Read the model definition and answer for the solid it produces. Units are mm, in the model's axes. Round coordinates to 2 decimals unless told otherwise and drop trailing zeros. Write each loop counter-clockwise with the first axis right and the second up, starting at its lowest first coordinate (ties: lowest second). Pieces come first, ordered by that corner, then holes.
from build123d import *

# Parameters (mm, degrees)
SKETCH1_R           = 3.175
BOSS_EXTRUDE1_DEPTH = 41.275
CUT_EXTRUDE5_DEPTH  = 83.672025196
CUT_EXTRUDE8_DEPTH  = 15.875


with BuildPart() as part:
    # Sketch1 → Boss-Extrude1 (new, symmetric)
    with BuildSketch(Plane(origin=(0, 0, 0), x_dir=(1, 0, 0), z_dir=(0, 1, 0))):
        with Locations(Location((0, 0, 0), (0, 0, 270))):
            Circle(SKETCH1_R)
    extrude(amount=BOSS_EXTRUDE1_DEPTH, both=True)

    # Sketch2 → Cut-Extrude5 (cut, through all)
    with BuildSketch(Plane(origin=(0, 41.275, 0), x_dir=(1, 0, 0), z_dir=(0, 1, 0))):
        with BuildLine():
            Line((-2.549322464, 1.892506268), (2.530677536, 1.917366999))
            ThreePointArc((2.530677536, 1.917366999), (-0.015537771, 3.174961981), (-2.549322464, 1.892506268))
        make_face()
    extrude(amount=-CUT_EXTRUDE5_DEPTH, mode=Mode.SUBTRACT)

    # Sketch5 → Cut-Extrude8 (cut)
    with BuildSketch(Plane(origin=(0, 41.275, 0), x_dir=(1, 0, 0), z_dir=(0, 1, 0))):
        with BuildLine():
            Line((2.530677536, 1.917366999), (-2.549322464, 1.892506268))
            ThreePointArc((-2.549322464, 1.892506268), (0.015537771, -3.174961981), (2.530677536, 1.917366999))
        make_face()
    extrude(amount=-CUT_EXTRUDE8_DEPTH, mode=Mode.SUBTRACT)


solid = part.part
Q1. Straight lines are drawn through the part: probe 1 along X at (y, z) = (0.5, 0.15); probe 2 along Z at (x, y) = (-0.25, 5); probe 3 along X at (y, z) = (-4.5, 1.85). For each, find the intervals that lie inside material, in ascending order.
Verdict:
probe 1: x = -3.17 to 3.17
probe 2: z = -1.9 to 3.17
probe 3: x = -2.58 to 2.58
Q2. Section B-B (z = 2.5) is taken. Determine the outline of the cut face in (x, y) (3 decimals), then the cut area to 3 significant figures.
Verdict:
outline: (-1.957, -41.275) - (1.957, -41.275) - (1.957, 25.4) - (-1.957, 25.4) - close
area: 261 mm2
Q3. Section C-C (x = 1.75) is taken. Determine the outline of the cut face in (y, z) (3 decimals), then the cut area to 3 significant figures.
Verdict:
outline: (-41.275, -1.914) - (25.4, -1.914) - (25.4, 2.649) - (-41.275, 2.649) - close
area: 304 mm2
